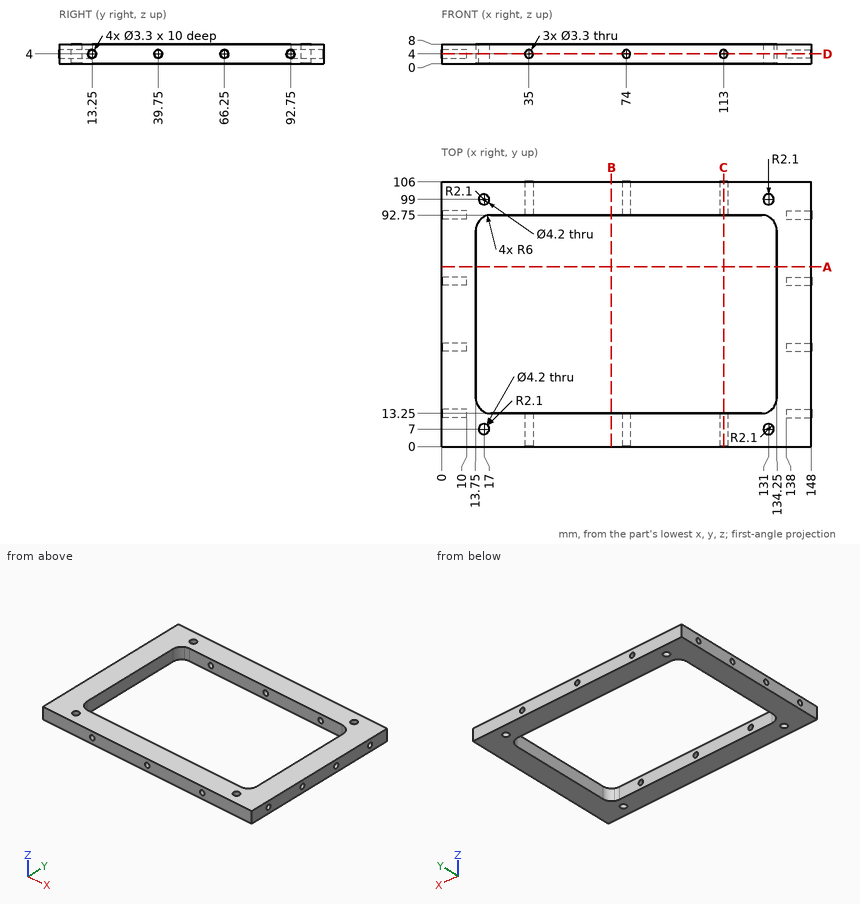
Part print with two shaded views. Sizes in mm from the minimum x, y, z corner. Coordinates: 2 decimals unless noted, no trailing zeros. Order: outer loops, then holes, each group sorted by start corner. A loop starts at its lowest first (then second) coordinate and runs counter-clockwise, first axis right, second up. Notation, with made-up numbers: (39, 85.5) - (88, 85.5) arc R18 cw to (88, 110.5) - close; hole circle Ø5 at (25.5, 77.25). An arc over 180 degrees is marked (long way). Write item = value, one per line. Start each with the question number.
1) Saw through at B-B on x = 68. Write the cut outline in (y, z), then the cut area to 3 significant figures.
2) Flat gauge pins, fed straight in: pin 1 Ø2.5 at (x, z) = (64, 5) entering from -Y; pin 2 Ø1 at (y, z) = (12.5, 4) entering from -X; pin 3 Ø1.6 at (y, z) = (40.5, 4) entering from +X. Where does each tip first touch, or does it go through?
3) Saw through at D-D on z = 4. Count the separate pieces of the cut face and the enclosed holes in it, then the cut area to 3 significant figures.
4) Saw through at C-C on x = 113. Write the cut outline in (y, z).
5) Wall check: line 1 along X through (y, z) = (9.75, 4); line 2 along Y through (x, z) = (5.5, 4); line 3 along X through (y, z) = (30.5, 5.75). Give the ranges that are in metal, low to high. Write a range as from..to.
6) Saw through at A-A on y = 72. Write the cut outline in (x, z), then the cut area to 3 significant figures.
From the geometry:
q1.outline = (0, 0) - (13.25, 0) - (13.25, 8) - (0, 8) - close; (92.75, 0) - (106, 0) - (106, 8) - (92.75, 8) - close
q1.area = 212 mm^2
q2.pin_1 = 0
q2.pin_2 = 10
q2.pin_3 = 138
q3.separate_pieces = 6
q3.enclosed_holes = 4
q3.area = 5,560 mm^2
q4.outline = (0, 0) - (13.25, 0) - (13.25, 2.35) - (0, 2.35) - close; (0, 5.65) - (13.25, 5.65) - (13.25, 8) - (0, 8) - close; (92.75, 0) - (106, 0) - (106, 2.35) - (92.75, 2.35) - close; (92.75, 5.65) - (106, 5.65) - (106, 8) - (92.75, 8) - close
q5.line_1 = 0..33.35, 36.65..72.35, 75.65..111.35, 114.65..148
q5.line_2 = 0..11.6, 14.9..38.1, 41.4..64.6, 67.9..91.1, 94.4..106
q5.line_3 = 0..13.75, 134.25..148
q6.outline = (0, 0) - (13.75, 0) - (13.75, 8) - (0, 8) - close; (134.25, 0) - (148, 0) - (148, 8) - (134.25, 8) - close
q6.area = 220 mm^2
